Geometry check sheet. Reference: the model listing, model coordinates, mm. Face numbers are marked on the shaded views. A direction names the side the tool comes from. Coordinates: 2 decimals unless noted, no trailing zeros. Order: outer loops, then holes, each group sorted by start corner. A loop starts at its lowest first (then second) coordinate and runs counter-clockwise, first axis right, second up. Notation, with made-up numbers: (5.25, 23.25) - (12.25, 23.25) arc R24 ccw to (12.25, 46.25) - close; hole circle Ø2 at (-19, 57). An arc over 180 degrees is marked (long way). Return JSON: item names as keys, results as strings. Group by question number.
Item 1: Scan lines: probe 1 along X at (y, z) = (25.4, 8.25); probe 2 along Y at (x, z) = (0, 9); probe 3 along Y at (x, z) = (3, 7.5). Record each from-to range of solid material in increasing order.
Item 2: Tool access check on the marked faces 5 and 6. Record the directions out of +Z, -Z, +X, -X, +Y, -Y that give a thin tool (end or side, any length) a straight path to the whole face; none if there is none.
Item 3: Section check C-C on x = -9.5. Enter the section's corners in (y, z), then the cut area to 3 significant figures.
Item 4: Gauge pin test, flat ends, axial feed: pin 1 (1.5 mm diameter, centred on y = -29, z = 1.5, fed in from -X); pin 2 (5 mm diameter, centred on y = 11, z = 5, fed in from -X). Record the tip position at first contact, or that the pin passes through.
Item 5: Section check D-D on z = 9.75. Enter the section's corners in (x, y).
Item 6: Draft check along X on the marked faces 1, 2, 3 and 4. Enter one of: pulls with the +X half, pulls with the -X half, needs draft (parallel to the pull), parting line crosses it, or undercut.
Item 7: Section check B-B on x = 0. Enter the section's corners in (y, z), then the cut area to 3 significant figures.
Item 8: Section check A-A on y = -25.4. Enter the section's corners in (x, z).
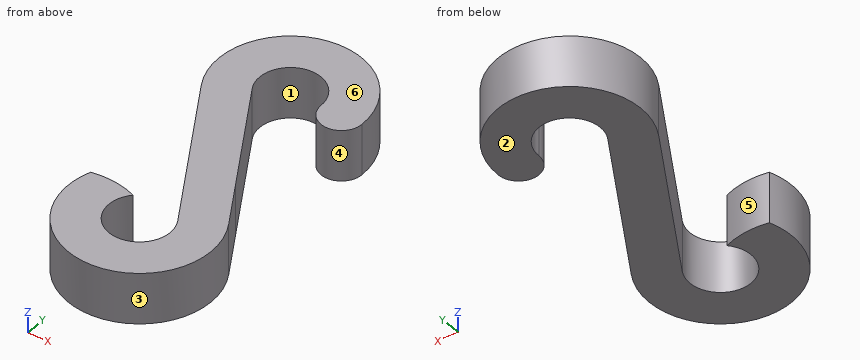
from build123d import *

# Parameters (mm, degrees)
F1_DEPTH = 12.7


with BuildPart() as f1:
    # F0 (on Top) → F1 (new body)
    with BuildSketch(Plane.XY):
        with BuildLine():
            ThreePointArc((17.778243, 25.150034), (-4.480962, 42.606086), (-15.397932, 16.51))
            Line((-15.397932, 16.51), (6.599114, -21.59))
            ThreePointArc((6.599114, -21.59), (-0.93735, -32.962128), (-5.469168, -20.094098))
            ThreePointArc((-5.469168, -20.094098), (-10.966834, -18.752892), (-16.616611, -19.074129))
            ThreePointArc((-16.616611, -19.074129), (1.419501, -43.123245), (15.397932, -16.51))
            Line((15.397932, -16.51), (8.832116, -5.137674))
            Line((8.832116, -5.137674), (-6.599114, 21.59))
            ThreePointArc((-6.599114, 21.59), (-1.869298, 32.787159), (7.617032, 25.187352))
            ThreePointArc((7.617032, 25.187352), (12.678979, 20.088088), (17.778243, 25.150034))
        make_face()
    extrude(amount=F1_DEPTH)


solid = f1.part
Computed:
{
 "1": {"probe 1": "x = -17.78 to -7.62, 7.62 to 17.78", "probe 2": "y = -43.18 to -33.02, -10.16 to 10.16, 33.02 to 43.18", "probe 3": "y = -42.93 to -32.4, -15.36 to 4.96, 32.4 to 42.93"},
 "2": {"face 5": "+Z, -Z", "face 6": "+Z, +X, -X, +Y, -Y"},
 "3": {"outline": "(-40.43, 0) - (-18.94, 0) - (-18.94, 12.7) - (-40.43, 12.7) - close; (6.29, 0) - (40.43, 0) - (40.43, 12.7) - (6.29, 12.7) - close", "area": "706 mm²"},
 "4": {"pin 1": "stops at x = -17.55", "pin 2": "stops at x = -13.66"},
 "5": {"outline": "(-16.62, -19.07) arc R17.78 ccw (long way) to (15.4, -16.51) - (-6.6, 21.59) arc R7.62 cw (long way) to (7.62, 25.19) arc R5.08 ccw to (17.78, 25.15) arc R17.78 ccw (long way) to (-15.4, 16.51) - (6.6, -21.59) arc R7.62 cw (long way) to (-5.47, -20.09) arc R19.18 ccw to start"},
 "6": {"face 1": "undercut", "face 2": "needs draft", "face 3": "parting line crosses it", "face 4": "undercut"},
 "7": {"outline": "(-43.18, 0) - (-33.02, 0) - (-33.02, 12.7) - (-43.18, 12.7) - close; (-10.16, 0) - (10.16, 0) - (10.16, 12.7) - (-10.16, 12.7) - close; (33.02, 0) - (43.18, 0) - (43.18, 12.7) - (33.02, 12.7) - close", "area": "516 mm²"},
 "8": {"outline": "(-17.78, 0) - (-7.62, 0) - (-7.62, 12.7) - (-17.78, 12.7) - close; (7.62, 0) - (17.78, 0) - (17.78, 12.7) - (7.62, 12.7) - close"}
}
